Design review of the part built by this model. Coordinates are the model's own, in mm. Give positions to 0.01 mm unless a question says otherwise; leave off trailing zeros. Order: outer loops, then holes, each group sorted by start corner. A loop starts at its lowest first (then second) coordinate and runs counter-clockwise, first axis right, second up. Notation, with made-up numbers: (35, -34.5) -> (94, -34.5) arc R30 cw to (94, -3.5) -> close; hole circle Ø5 at (1.5, -34.5). An arc over 180 degrees is marked (long way). One line per item, written item: value.
from build123d import *

# Parameters (mm, degrees)
SKETCH1_W                           = 50.8
SKETCH1_H                           = 50.8
BOSS_EXTRUDE1_DEPTH                 = 6.35
F_11_16_0_6875_DIAMETER_HOLE1_D     = 17.4625
F_11_16_0_6875_DIAMETER_HOLE1_DEPTH = 70.104
F_11_16_0_6875_DIAMETER_HOLE1_TIP   = 5.24626428
F_3_16_0_1875_DIAMETER_HOLE1_D      = 4.7625
F_3_16_0_1875_DIAMETER_HOLE1_DEPTH  = 70.104
F_3_16_0_1875_DIAMETER_HOLE1_TIP    = 1.430799349
F_29_0_136_DIAMETER_HOLE1_D         = 3.4544
F_29_0_136_DIAMETER_HOLE1_DEPTH     = 70.104
F_29_0_136_DIAMETER_HOLE1_TIP       = 1.037806461


with BuildPart() as part:
    # Sketch1 → Boss-Extrude1 (new body)
    with BuildSketch(Plane(origin=(0, 0, 0), x_dir=(0, 0, -1), z_dir=(1, 0, 0))):
        Rectangle(SKETCH1_W, SKETCH1_H)
    extrude(amount=BOSS_EXTRUDE1_DEPTH)

    # 11/16 (0.6875) Diameter Hole1
    with Locations(Plane(origin=(6.35, 0, 0), x_dir=(0, 0, -1), z_dir=(1, 0, 0))):
        with Locations((0, -13.97)):
            Hole(F_11_16_0_6875_DIAMETER_HOLE1_D / 2, depth=F_11_16_0_6875_DIAMETER_HOLE1_DEPTH)
            with Locations((0, 0, -(F_11_16_0_6875_DIAMETER_HOLE1_DEPTH + F_11_16_0_6875_DIAMETER_HOLE1_TIP / 2))):  # 118° drill point
                Cone(0, F_11_16_0_6875_DIAMETER_HOLE1_D / 2, F_11_16_0_6875_DIAMETER_HOLE1_TIP, mode=Mode.SUBTRACT)

    # 3/16 (0.1875) Diameter Hole1
    with Locations(Plane(origin=(6.35, 0, 0), x_dir=(0, 0, -1), z_dir=(1, 0, 0))):
        with Locations((0, 12.2301)):
            Hole(F_3_16_0_1875_DIAMETER_HOLE1_D / 2, depth=F_3_16_0_1875_DIAMETER_HOLE1_DEPTH)
            with Locations((0, 0, -(F_3_16_0_1875_DIAMETER_HOLE1_DEPTH + F_3_16_0_1875_DIAMETER_HOLE1_TIP / 2))):  # 118° drill point
                Cone(0, F_3_16_0_1875_DIAMETER_HOLE1_D / 2, F_3_16_0_1875_DIAMETER_HOLE1_TIP, mode=Mode.SUBTRACT)

    # #29 (0.136) Diameter Hole1
    with Locations(Plane(origin=(6.35, 0, 0), x_dir=(0, 0, -1), z_dir=(1, 0, 0))):
        with Locations((21, 12.2301), (-21, 11.74145915)):
            Hole(F_29_0_136_DIAMETER_HOLE1_D / 2, depth=F_29_0_136_DIAMETER_HOLE1_DEPTH)
            with Locations((0, 0, -(F_29_0_136_DIAMETER_HOLE1_DEPTH + F_29_0_136_DIAMETER_HOLE1_TIP / 2))):  # 118° drill point
                Cone(0, F_29_0_136_DIAMETER_HOLE1_D / 2, F_29_0_136_DIAMETER_HOLE1_TIP, mode=Mode.SUBTRACT)


solid = part.part
Item 1: Add section D-D on x = 1.25. Give the boundary of the cut face in (y, z).
Returned:
outline: (-25.4, -25.4) -> (25.4, -25.4) -> (25.4, 25.4) -> (-25.4, 25.4) -> close; hole circle Ø17.46 at (-13.97, 0); hole circle Ø4.76 at (12.23, 0); hole circle Ø3.45 at (11.74, 21); hole circle Ø3.45 at (12.23, -21)
Item 2: Add section A-A on z = 21. Give the boundary of the cut face in (x, y), plus the area to 3 significant figures.
Returned:
outline: (0, -25.4) -> (6.35, -25.4) -> (6.35, 10.01) -> (0, 10.01) -> close; (0, 13.47) -> (6.35, 13.47) -> (6.35, 25.4) -> (0, 25.4) -> close
area: 301 mm²
Item 3: Draft analysis for pull direction Z (two halves, no side actions). For faces 1 (the cylindrical face through (3.131, 13.943, -21.225)), 2 (the flat face through (3, 0, -25.4)), 3 (the flat face through (6.35, 0, 0)), state which applies: pulls with the +Z half, pulls with the -Z half, needs draft (parallel to the pull), parting line crosses it, or undercut.
Returned:
face 1: undercut
face 2: pulls with the -Z half
face 3: needs draft
Item 4: Add section B-B on y = -13.97. Give the boundary of the cut face in (x, z).
Returned:
outline: (0, -25.4) -> (6.35, -25.4) -> (6.35, -8.73) -> (0, -8.73) -> close; (0, 8.73) -> (6.35, 8.73) -> (6.35, 25.4) -> (0, 25.4) -> close
Item 5: Clearance check with flat-ended pins moving along their axes: P1, Ø4.5, axis at y = 12.23, z = 0, coming from the -X side; P2, Ø4, axis at y = 12.23, z = -21, coming from the +X side. State where each tip first meets the part, or that it passes through.
Returned:
P1: through
P2: x = 6.35
Item 6: To check wall thickness, follow line 1 along Y through (x, z) = (1.5, 0); line 2 along Y through (x, z) = (3.5, 21); line 3 along Y through (x, z) = (3.75, -2). State the ranges of each line that lie inside material, in increasing order. Write a range as from..to.
Returned:
line 1: -25.4..-22.7, -5.24..9.85, 14.61..25.4
line 2: -25.4..10.01, 13.47..25.4
line 3: -25.4..-22.47, -5.47..10.94, 13.52..25.4
Item 7: Add section C-C on z = 0. Give the boundary of the cut face in (x, y), plus the area to 3 significant figures.
Returned:
outline: (0, -25.4) -> (6.35, -25.4) -> (6.35, -22.7) -> (0, -22.7) -> close; (0, -5.24) -> (6.35, -5.24) -> (6.35, 9.85) -> (0, 9.85) -> close; (0, 14.61) -> (6.35, 14.61) -> (6.35, 25.4) -> (0, 25.4) -> close
area: 181 mm²
